from build123d import *

# Parameters (mm, degrees)
F1_DEPTH = 150
F2_W     = 20
F2_H     = 8
F2_R     = 3.4
F3_DEPTH = 300
F4_R     = 3


with BuildPart() as f1:
    # F0 (on Top) → F1 (new body, symmetric)
    with BuildSketch(Plane.XY):
        Polygon((30, 4), (30, 15), (19, 15), (19, 5), (11, 5), (11, 15), (-11, 15), (-11, 5), (-19, 5), (-19, 15), (-30, 15), (-30, 4), (-20, 4), (-20, -4), (-30, -4), (-30, -15), (-19, -15), (-19, -5), (-11, -5), (-11, -15), (11, -15), (11, -5), (19, -5), (19, -15), (30, -15), (30, -4), (20, -4), (20, 4), align=None)
    extrude(amount=F1_DEPTH, both=True)

    # F2 (on face) → F3 (cut)
    with BuildSketch(Plane.XY.offset(150)):
        Rectangle(F2_W, F2_H)
        with Locations((-15, 0)):
            Circle(F2_R)
        with Locations((15, 0)):
            Circle(F2_R)
    extrude(amount=-F3_DEPTH, mode=Mode.SUBTRACT)

    # F4
    f4_edges = [f1.edges().sort_by_distance(p)[0] for p in [
        (30, -15, 0),
        (30, 15, 0),
        (-30, -15, 0),
        (-30, 15, 0),
    ]]
    fillet(f4_edges, radius=F4_R)


solid = f1.part
Read the model definition and answer for the solid it produces. Units are mm, in the model's axes. A direction names the side the tool comes from. Coordinates: 2 decimals unless noted, no trailing zeros. Loops run counter-clockwise (first coordinate to the right, second up) from the corner with the lowest first, then second, coordinate; pieces in that order, holes last.
Q1. The part is cut by section A-A on x = -15. Write down the section's boundary in (y, z).
Q2. The part is cut by section C-C on x = 5. Write down the section's boundary in (y, z), and give its area (3 significant figures).
Q3. The mould has two halves that part along X. Classify faces 6 (the face through (-15, -5, 2)), 7 (the face through (30, 8, 2)), 8 (the face through (-25, 4, 2)): +X half, -X half, draft (parallel to the pull), parting line (faces both ways), or undercut.
Q4. Consider probe 1 along X at (y, z) = (-7.75, -106.5); probe 2 along Y at (x, z) = (-15, -69); probe 3 along Y at (x, z) = (7, -1.5). Determine where each line is inside the solid, lowest interval first.
Q5. Each of these flat-tipped pins is pushed along its axis until it touches: pin 1 Ø4 at (x, z) = (16.5, -21.5) entering from +Y; pin 2 Ø4 at (x, y) = (15, 0) entering from -Z (3 decimals); pin 3 Ø2.5 at (x, z) = (14, -35.5) entering from -Y. Where does it stop, or does it pass through?
Q6. The part is cut by section D-D on z = 112. Give the number of separate pieces and of enclosed holes in the cut face, and give its area (3 significant figures).
Q7. The part is cut by section B-B on y = 8.75. Write down the section's boundary in (x, z), and give its area (3 significant figures).
Q8. Which of the six approach directions +Z, -Z, +X, -X, +Y, -Y give full straight-line access (tool end or side, diameter ignored) to faces 1 (the face through (11, 10, 2)), 2 (the face through (20, 0, 2)), 3 (the face through (0, 4, 2)), 4 (the face through (-25, -4, 2)), 5 (the face through (15, -5, 2))?
Results below:
1. outline: (-5, -150) - (-3.4, -150) - (-3.4, 150) - (-5, 150) - close; (3.4, -150) - (5, -150) - (5, 150) - (3.4, 150) - close
2. outline: (-15, -150) - (-4, -150) - (-4, 150) - (-15, 150) - close; (4, -150) - (15, -150) - (15, 150) - (4, 150) - close
2. area: 6,600 mm2
3. face 6: undercut
3. face 7: +X half
3. face 8: draft
4. probe 1: x = -30 to -19, -11 to 11, 19 to 30
4. probe 2: y = -5 to -3.4, 3.4 to 5
4. probe 3: y = -15 to -4, 4 to 15
5. pin 1: stops at y = 5
5. pin 2: passes through
5. pin 3: stops at y = -5
6. separate pieces: 1
6. enclosed holes: 3
6. area: 1,080 mm2
7. outline: (-30, -150) - (-19, -150) - (-19, 150) - (-30, 150) - close; (-11, -150) - (11, -150) - (11, 150) - (-11, 150) - close; (19, -150) - (30, -150) - (30, 150) - (19, 150) - close
7. area: 13,200 mm2
8. face 1: +Z, -Z, +Y
8. face 2: +Z, -Z, +X
8. face 3: +Z, -Z
8. face 4: +Z, -Z, -X
8. face 5: +Z, -Z, -Y
